Autodesk Inventor part; units mm, degrees
ref_plane "YZ Plane" through (0, 0, 0) normal (1, 0, 0) x (0, 1, 0)
ref_plane "XZ Plane" through (0, 0, 0) normal (0, 1, 0) x (-1, 0, 0)
ref_plane "XY Plane" through (0, 0, 0) normal (0, 0, 1) x (1, 0, 0)
sketch "Sketch2" plane through (0, 0, 0) normal (0, 0, 1) x (1, 0, 0)
  line L0 (-110, 0) -> (110, 0) construction
  line L1 (-110, -90) -> (110, -90)
  line L2 (110, 90) -> (-110, 90)
  arc A0 (-110, 90) -> (-110, -90) centre (-110, 0) ccw
  arc A1 (110, -90) -> (110, 90) centre (110, 0) ccw
  line L3 (-200, 0) -> (200, 0) construction
  line L4 (-110, 140) -> (110, 140)
  arc A2 (110, -140) -> (110, 140) centre (110, 0) ccw
  line L5 (110, -140) -> (-110, -140)
  arc A3 (-110, 140) -> (-110, -140) centre (-110, 0) ccw
  point P0 (0, 0)
  dimension "Charging_hatch_width" = 400
  dimension "d11" = 400
  dimension "d12" = 180
  dimension "d13" = 50
extrude "Plate2" add sketch "Sketch2" along normal blind 8
sketch "Sketch3" plane through (0, 0, 8) normal (0, 0, 1) x (1, 0, 0)
  arc A0 (-110, 140) -> (-110, -140) centre (-110, 0) ccw construction
  line L0 (-110, 140) -> (110, 140) construction
  arc A1 (110, -140) -> (110, 140) centre (110, 0) ccw construction
  line L1 (110, -140) -> (-110, -140)
  circle A2 centre (-230, 0) radius 8.5
  arc A3 (-110, 120) -> (-110, -120) centre (-110, 0) ccw construction
  line L2 (-110, 120) -> (110, 120) construction
  arc A4 (110, -120) -> (110, 120) centre (110, 0) ccw construction
  line L3 (110, -120) -> (-110, -120) construction
  point P0 (0, 0)
  dimension "Charging_hatch_width" = 400
  dimension "d15" = 17
  dimension "d16" = 20
extrude "Cut1" cut sketch "Sketch3" against normal blind 8
pattern_circular "Circular Pattern1" count 5 over 180 about axis through (-110, 0, 0) along (0, 0, 1) of "Cut1" both ways yes
mirror "Mirror1" about plane through (0, 0, 0) normal (1, 0, 0) of "Cut1", "Circular Pattern1"
sketch "Sketch4" plane through (0, 0, 8) normal (0, 0, 1) x (1, 0, 0)
  circle A0 centre (-110, 120) radius 8.5 construction
  circle A1 centre (110, 120) radius 8.5 construction
  circle A2 centre (-110, -120) radius 8.5 construction
  circle A3 centre (110, -120) radius 8.5 construction
  circle A4 centre (0, -120) radius 8.5
  circle A5 centre (0, 120) radius 8.5
  point P0 (0, 0)
  dimension "Charging_hatch_width" = 400
  dimension "d22" = 0
extrude "Cut2" cut sketch "Sketch4" against normal blind 8
equation "\"d11\" = Charging_hatch_width"
equation "\"d12\" = Charging_hatch_hight"
equation "\"d17\" = Thickness"
equation "\"d23\" = Thickness"
equation "\"d14\" = Thickness"
equation "\"BendReliefWidth\" = Thickness"
equation "\"BendReliefDepth\" = 0.5 * Thickness"
equation "\"CornerReliefSize\" = 4 * Thickness"
equation "\"MinimumRemnant\" = 2 * Thickness"
equation "\"TransitionRadius\" = BendRadius"
equation "\"JacobiRadiusSize\" = BendRadius"
equation "\"GapSize\" = Thickness"
properties part number "PNS-631 charging flange" material "Steel"
CAD build for the part. Positions are in the model's coordinates, mm. A direction names the side the tool comes from. Round coordinates to 2 decimals unless told otherwise and drop trailing zeros. Write each loop counter-clockwise with the first axis right and the second up, starting at its lowest first coordinate (ties: lowest second). Pieces come first, ordered by that corner, then holes. Notation, with made-up numbers: M 77.5,-23.75 L 100.5,-23.75 A19 cw 100.5,10.25 Z; hole C -15.75,72.25 d5. An arc over 180 degrees is marked long. Use a Markdown table: item, result. Add a question column.
1. Slice it at A-A on x = 0. Give the cut face in (y, z).
2. 3-axis set-ups, long thin cutter, end or side, ignore diameter. For faces 5 (the face through (-3, 95, 8)), 6 (the face through (199.98, 1.98, 3.94)): which of +Z, -Z, +X, -X, +Y, -Y reach the whole face in a straight line?
3. Slice it at C-C on z = 3.25. Give the number of separate pieces and of enclosed holes in the cut face, then the cut area to 3 significant figures.
4. Slice it at B-B on y = 31. Give the cut face in (x, z).
5. Flat gauge pins, fed straight in: P1, Ø19.5, axis at x = -194.85, y = -84.85, coming from the -Z side; P2, Ø13.5, axis at x = 194.85, y = 84.85, coming from the +Z side; P3, Ø1.5, axis at x = 180.5, z = 2, coming from the -Y side; P4, Ø2, axis at y = -35, z = 1.5, coming from the -X side. Where does each tip first touch, or does it go through?
6. Drill centre lines: probe 1 along X at (y, z) = (117.5, 5); probe 2 along X at (y, z) = (-2, 3); probe 3 along Y at (x, z) = (92.5, 2). Where is each one in solid material? Low to high.
7. Pull direction X, two halves, no side cores. Call faces 1 (the face through (238.49, -0.37, 4.06)), 2 (the face through (-249.966, -3.079, 3.944)), 3 (the face through (187, 81.6, 4.1)), 4 (the face through (249.966, 3.079, 3.944)): released by +X, released by -X, zero draft, split by the parting line, or undercut.
8. Slice it at D-D on x = 90.5. Give the cut face in (y, z), then the cut area to 3 significant figures.
Reply:
| question | item | result |
|---|---|---|
| 1 | outline | M -140,0 L -128.5,0 L -128.5,8 L -140,8 Z; M -111.5,0 L -90,0 L -90,8 L -111.5,8 Z; M 90,0 L 111.5,0 L 111.5,8 L 90,8 Z; M 128.5,0 L 140,0 L 140,8 L 128.5,8 Z |
| 2 | face 5 | +Z, +X, -X, +Y, -Y |
| 2 | face 6 | +Z, -Z |
| 3 | separate pieces | 1 |
| 3 | enclosed holes | 13 |
| 3 | area | 55,400 mm^2 |
| 4 | outline | M -246.52,0 L -194.49,0 L -194.49,8 L -246.52,8 Z; M 194.49,0 L 246.52,0 L 246.52,8 L 194.49,8 Z |
| 5 | P1 | stops at z = 0 |
| 5 | P2 | passes through |
| 5 | P3 | stops at y = -121.39 |
| 5 | P4 | stops at x = -245.81 |
| 6 | probe 1 | x = -186.12 to -118.12, -101.88 to -8.12, 8.12 to 101.88, 118.12 to 186.12 |
| 6 | probe 2 | x = -249.99 to -238.26, -221.74 to -199.98, 199.98 to 221.74, 238.26 to 249.99 |
| 6 | probe 3 | y = -140 to -90, 90 to 140 |
| 7 | face 1 | undercut |
| 7 | face 2 | released by -X |
| 7 | face 3 | undercut |
| 7 | face 4 | released by +X |
| 8 | outline | M -140,0 L -90,0 L -90,8 L -140,8 Z; M 90,0 L 140,0 L 140,8 L 90,8 Z |
| 8 | area | 800 mm^2 |
